from build123d import *
from OCP.BRepFilletAPI import BRepFilletAPI_MakeChamfer

# Parameters (mm, degrees)
BOSS_EXTRUDE1_DEPTH             = 1
BOSS_EXTRUDE2_REACH             = 42.227
SKETCH2_W                       = 19.144631242
SKETCH2_H                       = 6
BOSS_EXTRUDE2_DIRECTION_2_DEPTH = 10
CUT_EXTRUDE1_DEPTH              = 8
CUT_EXTRUDE2_DEPTH              = 40.207813431
CUT_EXTRUDE2_DEPTH_BACK         = 40.207813431
SKETCH4_W                       = 8
SKETCH4_H                       = 2
CHAMFER1_SIZE                   = 2
CHAMFER2_SIZE                   = 10
CHAMFER2_SIZE2                  = 5.773502692
FILLET1_START                   = -1
FILLET1_DEPTH                   = 3
FILLET1_2_DEPTH                 = 2
BOSS_EXTRUDE3_START             = -6
SKETCH5_W                       = 10
SKETCH5_H                       = 1.6
BOSS_EXTRUDE3_DEPTH             = 10.5


with BuildPart() as part:
    # Sketch1 → Boss-Extrude1 (new, symmetric)
    with BuildSketch(Plane(origin=(0, 0, 0), x_dir=(1, 0, 0), z_dir=(0, 1, 0))):
        Polygon((-8, 0), (0, 0), (0, -1.6), (-9.572315621, -1.6), (-9.800648012, 11.481153904), (-12.360970922, 15.137673965), (-22.096439397, 32), (-20.248918536, 32), (-11.01025903, 15.998172342), (-8.209428877, 11.998172342), align=None)
    boss_extrude1 = extrude(amount=BOSS_EXTRUDE1_DEPTH, both=True)

    # Mirror1: Boss-Extrude1 across plane
    add(boss_extrude1.mirror(Plane(origin=(0, 1, 0), x_dir=(0, 0, 1), z_dir=(-1, 0, 0))))

    # Boss-Extrude2: up to this face of the body (flat: up to its plane)
    boss_extrude2_end = Plane(part.part.faces().sort_by_distance((0, 0, 0))[0])
    # Sketch2 → Boss-Extrude2 (add, up to the picked face)
    with BuildSketch(Plane.XY.offset(1.6), mode=Mode.PRIVATE) as boss_extrude2_sk1:
        with Locations((0, -2)):
            Rectangle(SKETCH2_W, SKETCH2_H)
    boss_extrude2_tool1 = split(extrude(boss_extrude2_sk1.sketch, amount=-BOSS_EXTRUDE2_REACH, mode=Mode.PRIVATE), bisect_by=boss_extrude2_end, keep=Keep.BOTH, mode=Mode.PRIVATE)
    add(boss_extrude2_tool1.solids().sort_by(Axis((0, -2, 1.6), (0, 0, -1)))[0])

    # Sketch2 → Boss-Extrude2 direction 2 (add)
    with BuildSketch(Plane.XY.offset(1.6)):
        with Locations((0, -2)):
            Rectangle(SKETCH2_W, SKETCH2_H)
    extrude(amount=BOSS_EXTRUDE2_DIRECTION_2_DEPTH)

    # Sketch3 → Cut-Extrude1 (cut)
    with BuildSketch(Plane.XY.offset(11.6)):
        with BuildLine():
            Line((-1.5, 0.826658805), (-1.5, 1))
            Line((-1.5, 1), (1.5, 1))
            Line((1.5, 1), (1.5, 0.826658805))
            ThreePointArc((1.5, 0.826658805), (3.2, -2), (1.5, -4.826658805))
            Line((1.5, -4.826658805), (1.5, -5))
            Line((1.5, -5), (-1.5, -5))
            Line((-1.5, -5), (-1.5, -4.826658805))
            ThreePointArc((-1.5, -4.826658805), (-3.2, -2), (-1.5, 0.826658805))
        make_face()
    extrude(amount=-CUT_EXTRUDE1_DEPTH, mode=Mode.SUBTRACT)

    # Sketch4 → Cut-Extrude2 (cut, two sides: drawn at the far end of the back side and taken through both)
    with BuildSketch(Plane(origin=(0, 0, 0), x_dir=(1, 0, 0), z_dir=(0, 1, 0)).offset(-CUT_EXTRUDE2_DEPTH_BACK)):
        with Locations((0, -4.6)):
            Rectangle(SKETCH4_W, SKETCH4_H)
    extrude(amount=CUT_EXTRUDE2_DEPTH + CUT_EXTRUDE2_DEPTH_BACK, mode=Mode.SUBTRACT)

    # Chamfer1
    chamfer1_edges = [part.edges().sort_by_distance(p)[0] for p in [
        (-8.78615781, -1, 0),
        (8.78615781, -1, 0),
    ]]
    chamfer(chamfer1_edges, length=CHAMFER1_SIZE)

    # Chamfer2: one chamfer whose edges measure the first distance from different faces: ONE call of the kernel's chamfer builder (chamfer() names one face for all edges)
    chamfer2_edges_1 = [part.edges().sort_by_distance(p)[0] for p in [
        (9.572315621, -2, 11.6),
    ]]
    chamfer2_side_1 = [part.faces().sort_by_distance(p)[0] for p in [
        (9.572315621, -2.083820663, 5.844834308),
    ]]
    chamfer2_edges_2 = [part.edges().sort_by_distance(p)[0] for p in [
        (-9.572315621, -2, 11.6),
    ]]
    chamfer2_side_2 = [part.faces().sort_by_distance(p)[0] for p in [
        (-9.572315621, -2.083820663, 5.844834308),
    ]]
    chamfer2 = BRepFilletAPI_MakeChamfer(part.part.solid().wrapped)
    for e in chamfer2_edges_1:
        chamfer2.Add(CHAMFER2_SIZE, CHAMFER2_SIZE2, e.wrapped, chamfer2_side_1[0].wrapped)  # the first distance lies on this face
    for e in chamfer2_edges_2:
        chamfer2.Add(CHAMFER2_SIZE, CHAMFER2_SIZE2, e.wrapped, chamfer2_side_2[0].wrapped)  # the first distance lies on this face
    add(Compound.cast(chamfer2.Shape()), mode=Mode.REPLACE)

    # Fillet1: read off the stored shape, not the designer's step
    # Fillet1 outline → Fillet1 (cut)
    with BuildSketch(Plane(origin=(0, 0, 0), x_dir=(1, 0, 0), z_dir=(0, 1, 0)).offset(FILLET1_START)):
        with BuildLine():
            Line((12.360970922, 15.137673965), (12.622936579, 15.591411793))
            ThreePointArc((12.622936579, 15.591411793), (12.351329084, 15.143816493), (12.060456265, 14.708494557))
            Line((12.060456265, 14.708494557), (12.360970922, 15.137673965))
        make_face()
        with BuildLine():
            ThreePointArc((8.145400044, 8.329962936), (8.73089419, 11.828737991), (10.313747854, 15.003451295))
            Line((10.313747854, 15.003451295), (8.209428877, 11.998172342))
            Line((8.209428877, 11.998172342), (8.145400044, 8.329962936))
        make_face()
        with BuildLine():
            Line((-12.360970922, 15.137673965), (-12.060456265, 14.708494557))
            ThreePointArc((-12.060456265, 14.708494557), (-12.351329084, 15.143816493), (-12.622936579, 15.591411793))
            Line((-12.622936579, 15.591411793), (-12.360970922, 15.137673965))
        make_face()
        with BuildLine():
            Line((-8.209428877, 11.998172342), (-10.313747854, 15.003451295))
            ThreePointArc((-10.313747854, 15.003451295), (-8.73089419, 11.828737991), (-8.145400044, 8.329962936))
            Line((-8.145400044, 8.329962936), (-8.209428877, 11.998172342))
        make_face()
    extrude(amount=FILLET1_DEPTH, mode=Mode.SUBTRACT)

    # Fillet1 2 outline → Fillet1 2 (add)
    with BuildSketch(Plane(origin=(0, 0, 0), x_dir=(1, 0, 0), z_dir=(0, 1, 0)).offset(FILLET1_START)):
        with BuildLine():
            ThreePointArc((9.736619178, 7.812944498), (10.322113325, 11.311719553), (11.904966989, 14.486432857))
            Line((11.904966989, 14.486432857), (9.800648012, 11.481153904))
            Line((9.800648012, 11.481153904), (9.736619178, 7.812944498))
        make_face()
        with BuildLine():
            ThreePointArc((11.272224688, 16.45191017), (11.000617192, 16.00431487), (10.709744374, 15.568992934))
            Line((10.709744374, 15.568992934), (11.01025903, 15.998172342))
            Line((11.01025903, 15.998172342), (11.272224688, 16.45191017))
        make_face()
        with BuildLine():
            Line((-9.800648012, 11.481153904), (-11.904966989, 14.486432857))
            ThreePointArc((-11.904966989, 14.486432857), (-10.322113325, 11.311719553), (-9.736619178, 7.812944498))
            Line((-9.736619178, 7.812944498), (-9.800648012, 11.481153904))
        make_face()
        with BuildLine():
            ThreePointArc((-10.709744374, 15.568992934), (-11.000617192, 16.00431487), (-11.272224688, 16.45191017))
            Line((-11.272224688, 16.45191017), (-11.01025903, 15.998172342))
            Line((-11.01025903, 15.998172342), (-10.709744374, 15.568992934))
        make_face()
    extrude(amount=FILLET1_2_DEPTH)

    # Sketch5 → Boss-Extrude3 (add)
    with BuildSketch(Plane.XZ.offset(5).offset(BOSS_EXTRUDE3_START)):
        with Locations((0, 0.8)):
            Rectangle(SKETCH5_W, SKETCH5_H)
    extrude(amount=BOSS_EXTRUDE3_DEPTH)


solid = part.part
Input: part model. Units: mm. Frame: model coordinates. A direction names the side the tool comes from. Give positions to 0.01 mm unless a question says otherwise; leave off trailing zeros. Order: outer loops, then holes, each group sorted by start corner. A loop starts at its lowest first (then second) coordinate and runs counter-clockwise, first axis right, second up. Notation, with made-up numbers: M 62,3 L 119,3 A16 ccw 119,12 Z; hole C 63.25,82 d1. An arc over 180 degrees is marked long. Answer as a JSON object with one key per item and string values.
1. First-contact query: P1, Ø7, axis at x = -13, z = -16.5, coming from the -Y side; P2, Ø3, axis at x = -3, y = -1, coming from the -Z side; P3, Ø1.5, axis at x = -0.5, y = -7.5, coming from the +Z side. Flat tips, straight axial feed; report the tip coordinate or a pass-through.
Result sheet:
{"P1": "y = -1", "P2": "z = 0", "P3": "z = 1.6"}
2. Reachability of faces 1 (the flat face through (-4, -2, 5)), 2 (the cylindrical face through (10.307, -0.014, -11.264)), 3 (the flat face through (15.82, 0.01, -24.33)), 4 (the flat face through (9.572, -3, 1)) from +Z, -Z, +X, -X, +Y, -Y: full face, straight path, thin tool, end or side. Return the list, or none.
Result sheet:
{"face 1": "+Y, -Y", "face 2": "+Z, +X, +Y, -Y", "face 3": "-Z, +Y, -Y", "face 4": "+Z, -Z, +X, -Y"}
3. Cut plane A-A, the plane z = -21. Output: boundary loops of the cut face in (x, y).
Result sheet:
{"outline": "M -15.75,-1 L -13.9,-1 L -13.9,1 L -15.75,1 Z; M 13.9,-1 L 15.75,-1 L 15.75,1 L 13.9,1 Z"}
4. Cut plane B-B, the plane y = -2.25. Output: boundary loops of the cut face in (x, z).
Result sheet:
{"outline": "M -9.57,-0.75 L -8.01,-0.75 L -8,0 L 8,0 L 8.01,-0.75 L 9.57,-0.75 L 9.57,1.6 L 3.8,11.6 L 3.19,11.6 L 3.19,5.6 L 4,5.6 L 4,3.6 L -4,3.6 L -4,5.6 L -3.19,5.6 L -3.19,11.6 L -3.8,11.6 L -9.57,1.6 Z"}
5. Ray query, line 1 (Z direction, x = 1, y = 0.5); line 2 (X direction, y = 0, z = -3.5); line 3 (Z direction, x = -5, y = -4.75). Return the intervals inside material, ascending. Write a range as [from, to].
Result sheet:
{"line 1": "[0, 3.6]", "line 2": "[-9.66, -8.06], [8.06, 9.66]", "line 3": "[0, 9.52]"}
6. Pull-direction query (Y, two-part tool) for faces 5 (the cylindrical face through (-10.34, -0.01, -11.36)), 6 (the flat face through (13, -1, -18)), 7 (the cylindrical face through (3.2, -2, 8.6)), 8 (the flat face through (-2, 1, 1)); classes: +Y half, -Y half, draft (parallel to the pull), parting line (faces both ways), or undercut.
Result sheet:
{"face 5": "draft", "face 6": "-Y half", "face 7": "undercut", "face 8": "+Y half"}
7. Cut plane D-D, the plane z = 7. Output: boundary loops of the cut face in (x, y), and give its area (3 significant figures).
Result sheet:
{"outline": "M -6.45,-5 L -1.5,-5 L -1.5,-4.83 A3.2 cw -1.5,0.83 L -1.5,1 L -6.45,1 Z; M 1.5,-5 L 6.45,-5 L 6.45,1 L 1.5,1 L 1.5,0.83 A3.2 cw 1.5,-4.83 Z", "area": "45.8 mm²"}
